```python
from build123d import *

# Parameters (mm, degrees)
F0_R     = 37.5
F1_DEPTH = 10
F2_W     = 9.3
F2_H     = 49.5
F3_DEPTH = 8
F2_R     = 10
F4_DEPTH = 10.001


with BuildPart() as f1:
    # F0 (on Top) → F1 (new body)
    with BuildSketch(Plane.XY):
        Circle(F0_R)
    extrude(amount=F1_DEPTH)

    # F2 (on face) → F3 (cut)
    with BuildSketch(Plane.XY.offset(10)):
        with Locations((-19.65, 0)):
            Rectangle(F2_W, F2_H)
        with Locations((19.65, 0)):
            Rectangle(F2_W, F2_H)
    extrude(amount=-F3_DEPTH, mode=Mode.SUBTRACT)

    # F2 (on face) → F4 (cut, through all)
    with BuildSketch(Plane.XY.offset(10)):
        with Locations((0, 24)):
            Circle(F2_R)
        Circle(F2_R)
        with Locations((0, -24)):
            Circle(F2_R)
    extrude(amount=-F4_DEPTH, mode=Mode.SUBTRACT)


solid = f1.part
```
Can you work these out from the model? Positions are in its coordinate system, mm. A direction names the side the tool comes from. Give positions to 0.01 mm unless a question says otherwise; leave off trailing zeros. Loops run counter-clockwise (first coordinate to the right, second up) from the corner with the lowest first, then second, coordinate; pieces in that order, holes last. Notation, with made-up numbers: M 41,16 L 84,16 A20 ccw 84,26 Z; hole C 36,-32.75 d5. An arc over 180 degrees is marked long. Use one line per item in the form item = value. Start each with the question number.
(1) Thinking about a two-plate mould opening in X: for faces 1 (the flat face through (8, -8, 0)), 2 (the flat face through (15, 0, 6)), 3 (the cylindrical face through (-4.88, 37.18, 4.93)), 4 (the flat face through (-20, 0, 2)), which applies, released by +X, released by -X, zero draft, split by the parting line, or undercut?
(2) I want a section at A-A, the plane y = 0. Write out the boundary of the cut face in (x, z).
(3) Please list where these lines run through material, in increasing order: line 1 (Y direction, x = 0.5, z = 3); line 2 (X direction, y = -21.5, z = 3); line 3 (X direction, y = -21, z = 3.75).
(4) I want a section at D-D, the plane y = -13. Write out the boundary of the cut face in (x, z), and give its area (3 significant figures).
(5) I'm going to push flat-ended pins straight in: P1, Ø1.5, axis at y = -10, z = 8, coming from the +X side; P2, Ø4, axis at x = 18, z = 6, coming from the -Y side; P3, Ø2.5, axis at x = -20, z = 7, coming from the -Y side. Where does each tip first touch, or does it pass through?
(6) On a 3-axis mill with a long thin cutter (end or side, diameter ignored), from which of +Z, -Z, +X, -X, +Y, -Y can I reach the whole of each face in a straight line? I mean faces 5 (the flat face through (-20, 24.75, 6)), 6 (the flat face through (8, -8, 10)). Say none if no direction works.
(7) I want a section at B-B, the plane z = 7.75. Write out the boundary of the cut face in (x, y), and give its area (3 significant figures).
(8) I want a section at C-C, the plane x = 0. Write out the boundary of the cut face in (y, z), and give its area (3 significant figures).
Worked out:
q1.face_1 = zero draft
q1.face_2 = undercut
q1.face_3 = split by the parting line
q1.face_4 = undercut
q2.outline = M -37.5,0 L -10,0 L -10,10 L -15,10 L -15,2 L -24.3,2 L -24.3,10 L -37.5,10 Z; M 10,0 L 37.5,0 L 37.5,10 L 24.3,10 L 24.3,2 L 15,2 L 15,10 L 10,10 Z
q3.line_1 = -37.5 to -33.99, -14.01 to -9.99, 9.99 to 14.01, 33.99 to 37.5
q3.line_2 = -30.72 to -24.3, -15 to -9.68, 9.68 to 15, 24.3 to 30.72
q3.line_3 = -31.07 to -24.3, -15 to -9.54, 9.54 to 15, 24.3 to 31.07
q4.outline = M -35.17,0 L 35.17,0 L 35.17,10 L 24.3,10 L 24.3,2 L 15,2 L 15,10 L -15,10 L -15,2 L -24.3,2 L -24.3,10 L -35.17,10 Z
q4.area = 555 mm²
q5.P1 = 36.34
q5.P2 = -33.92
q5.P3 = -32.48
q6.face_5 = +Z
q6.face_6 = +Z, +X, -X, +Y, -Y
q7.outline = C 0,0 d75; hole M -24.3,-24.75 L -15,-24.75 L -15,24.75 L -24.3,24.75 Z; hole C 0,-24 d20; hole C 0,0 d20; hole C 0,24 d20; hole M 15,-24.75 L 24.3,-24.75 L 24.3,24.75 L 15,24.75 Z
q7.area = 2,550 mm²
q8.outline = M -37.5,0 L -34,0 L -34,10 L -37.5,10 Z; M -14,0 L -10,0 L -10,10 L -14,10 Z; M 10,0 L 14,0 L 14,10 L 10,10 Z; M 34,0 L 37.5,0 L 37.5,10 L 34,10 Z
q8.area = 150 mm²
